Geometry check sheet. Reference: the model listing, model coordinates, mm. Round coordinates to 2 decimals unless told otherwise and drop trailing zeros. Write each loop counter-clockwise with the first axis right and the second up, starting at its lowest first coordinate (ties: lowest second). Pieces come first, ordered by that corner, then holes. Notation, with made-up numbers: M -10.5,-1.75 L 43.5,-1.75 A27 cw 43.5,18.25 Z; hole C 55,57 d11. An arc over 180 degrees is marked long. Use a Markdown table: item, result.
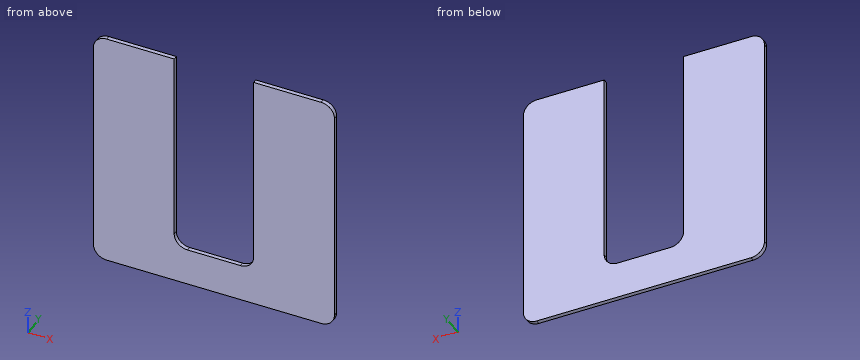
```python
from build123d import *

# Parameters (mm, degrees)
SKETCH1_W           = 91
SKETCH1_H           = 91
BOSS_EXTRUDE1_DEPTH = 1.6
SKETCH2_W           = 30
SKETCH2_H           = 77
CUT_EXTRUDE1_DEPTH  = 65.366606249
FILLET1_R           = 5


with BuildPart() as part:
    # Sketch1 → Boss-Extrude1 (new body)
    with BuildSketch(Plane(origin=(0, 0, 0), x_dir=(1, 0, 0), z_dir=(0, 1, 0))):
        Rectangle(SKETCH1_W, SKETCH1_H)
    extrude(amount=BOSS_EXTRUDE1_DEPTH)

    # Sketch2 → Cut-Extrude1 (cut, through all)
    with BuildSketch(Plane(origin=(0, 1.6, 0), x_dir=(1, 0, 0), z_dir=(0, 1, 0))):
        with Locations((0, -7)):
            Rectangle(SKETCH2_W, SKETCH2_H)
    extrude(amount=-CUT_EXTRUDE1_DEPTH, mode=Mode.SUBTRACT)

    # Fillet1
    fillet1_edges = [part.edges().sort_by_distance(p)[0] for p in [
        (15, 0.8, -31.5),
        (-15, 0.8, -31.5),
        (-45.5, 0.8, 45.5),
        (45.5, 0.8, 45.5),
        (45.5, 0.8, -45.5),
        (-45.5, 0.8, -45.5),
    ]]
    fillet(fillet1_edges, radius=FILLET1_R)


solid = part.part
```
Item 1: Material ranges on line 1 along X through (y, z) = (0.3, 10); line 2 along Z through (x, y) = (-10, 0.45); line 3 along Z through (x, y) = (-14, 0.8), recorded low to high. Write a range as from..to.
Outcome:
| item | result |
|---|---|
| line 1 | x = -45.5..-15, 15..45.5 |
| line 2 | z = -45.5..-31.5 |
| line 3 | z = -45.5..-29.5 |
Item 2: Cross-section at B-B, the plane y = 0.75. Record the cut outline in (x, z).
Outcome:
| item | result |
|---|---|
| outline | M -45.5,-40.5 A5 ccw -40.5,-45.5 L 40.5,-45.5 A5 ccw 45.5,-40.5 L 45.5,40.5 A5 ccw 40.5,45.5 L 15,45.5 L 15,-26.5 A5 cw 10,-31.5 L -10,-31.5 A5 cw -15,-26.5 L -15,45.5 L -40.5,45.5 A5 ccw -45.5,40.5 Z |
Item 3: Cross-section at A-A, the plane z = 16. Record the cut outline in (x, y), and give its area (3 significant figures).
Outcome:
| item | result |
|---|---|
| outline | M -45.5,0 L -15,0 L -15,1.6 L -45.5,1.6 Z; M 15,0 L 45.5,0 L 45.5,1.6 L 15,1.6 Z |
| area | 97.6 mm2 |
Item 4: Cross-section at C-C, the plane x = 12. Record the cut outline in (y, z), and give its area (3 significant figures).
Outcome:
| item | result |
|---|---|
| outline | M 0,-45.5 L 1.6,-45.5 L 1.6,-31.08 L 0,-31.08 Z |
| area | 23.1 mm2 |
